from build123d import *

# Parameters (mm, degrees)
F1_DEPTH = 147.066
F2_T     = -50.8


with BuildPart() as f1:
    # F0 (on Front) → F1 (new body)
    with BuildSketch(Plane.XZ):
        Polygon((-87.962036, -7.561638), (-62.522302, -62.333458), (-7.827687, -87.93876), (50.529589, -72.396539), (85.243509, -22.979173), (80.071044, 37.190404), (37.432448, 79.958177), (-22.721207, 85.312631), (-72.243357, 50.748356), align=None)
    extrude(amount=F1_DEPTH)

    # F2
    f2_openings = [f1.faces().sort_by_distance(p)[0] for p in [
        (0, -147.066, 0),
    ]]
    offset(amount=F2_T, openings=f2_openings)


solid = f1.part
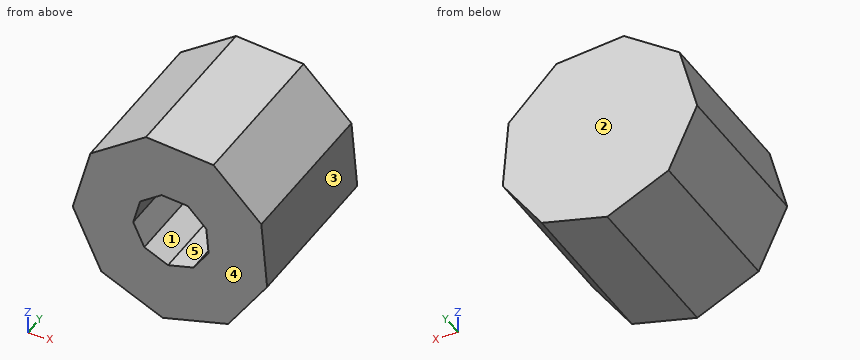
Can you work these out from the model? Positions are in its coordinate system, mm. Face numbers are marked on the shaded views. A direction names the side the tool comes from. Coordinates: 2 decimals unless noted, no trailing zeros. Loops run counter-clockwise (first coordinate to the right, second up) from the corner with the lowest first, then second, coordinate; pieces in that order, holes last. Notation, with made-up numbers: M 88,-38.75 L 109,-38.75 A26 ccw 109,-18.75 Z; hole C -26.75,2 d7. An arc over 180 degrees is marked long. Return JSON: item names as keys, results as strings. Group by question number.
Item 1: On a 3-axis mill with a long thin cutter (end or side, diameter ignored), from which of +Z, -Z, +X, -X, +Y, -Y can I reach the whole of each face in a straight line? I mean the marked faces 4 and 5. Say none if no direction works.
Item 2: I'm going to push flat-ended pins straight in: pin 1 Ø20 at (x, z) = (-2.5, -1.5) entering from -Y; pin 2 Ø8 at (x, y) = (-31.5, -111.5) entering from -Z; pin 3 Ø1.5 at (x, y) = (-6, -114) entering from +Z. Where does each tip first touch, or does it pass through?
Item 3: Imagine slicing it at C-C (y = -47). Please give me the cut outline in (x, z), and give its area (3 significant figures).
Item 4: Imagine slicing it at D-D (z = -15.5). Please give me the cut outline in (x, y).
Item 5: Imagine slicing it at B-B (x = 24). Please give me the cut outline in (y, z), and give its area (3 significant figures).
Item 6: If I drill on L1, parallel to Y at x = -7.5, z = -23; L2, parallel to X at y = -134, z = 6; L3, parallel to X at y = -124, z = -17, over which ranges is the centre line in solid material (lowest first)? Write a range as from..to.
Item 7: Imagine slicing it at A-A (y = -82). Please give me the cut outline in (x, z).
Item 8: Thinking about a two-plate mould opening in X: for the marked faces 1, 2 and 3, which applies, released by +X, released by -X, zero draft, split by the parting line, or undercut?
Verdict:
{
 "1": {"face 4": "+Z, -Z, +X, -X, -Y", "face 5": "-Y"},
 "2": {"pin 1": "stops at y = -50.8", "pin 2": "stops at z = -78.73", "pin 3": "stops at z = 83.89"},
 "3": {"outline": "M -87.96,-7.56 L -62.52,-62.33 L -7.83,-87.94 L 50.53,-72.4 L 85.24,-22.98 L 80.07,37.19 L 37.43,79.96 L -22.72,85.31 L -72.24,50.75 Z", "area": "22,500 mm^2"},
 "4": {"outline": "M -84.27,-147.07 L -28.26,-147.07 L -28.26,-50.8 L 28.42,-50.8 L 28.42,-147.07 L 84.6,-147.07 L 84.6,0 L -84.27,0 Z"},
 "5": {"outline": "M -147.07,-79.46 L 0,-79.46 L 0,81.15 L -147.07,81.15 L -147.07,21.48 L -50.8,21.48 L -50.8,-21.79 L -147.07,-21.79 Z", "area": "19,500 mm^2"},
 "6": {"L1": "y = -50.8..0", "L2": "x = -84.31..-31.69, 31.76..82.75", "L3": "x = -83.58..-27.57, 27.36..84.73"},
 "7": {"outline": "M -87.96,-7.56 L -62.52,-62.33 L -7.83,-87.94 L 50.53,-72.4 L 85.24,-22.98 L 80.07,37.19 L 37.43,79.96 L -22.72,85.31 L -72.24,50.75 Z; hole M -34.1,-2.93 L -24.24,-24.16 L -3.03,-34.09 L 19.59,-28.07 L 33.05,-8.91 L 31.04,14.42 L 14.51,31 L -8.81,33.07 L -28.01,19.67 Z"},
 "8": {"face 1": "undercut", "face 2": "zero draft", "face 3": "released by +X"}
}
